Autodesk Inventor part; units mm, degrees
ref_plane "YZ Plane" through (0, 0, 0) normal (1, 0, 0) x (0, 1, 0)
ref_plane "XZ Plane" through (0, 0, 0) normal (0, 1, 0) x (-1, 0, 0)
ref_plane "XY Plane" through (0, 0, 0) normal (0, 0, 1) x (1, 0, 0)
sketch "Sketch1" plane through (0, 0, 0) normal (0, 1, 0) x (-1, 0, 0)
  circle A0 centre (0, 0) radius 50
  circle A1 centre (0, 0) radius 40
  line L0 (50, 0) -> (-50, 0)
  line L1 (-50, 0) -> (-50, 50)
  line L2 (-50, 50) -> (50, 50)
  line L3 (50, 50) -> (50, 0)
  line L4 (6, -46) -> (-6, -46)
  line L5 (-6, -46) -> (-6, -62)
  line L6 (-6, -62) -> (6, -62)
  line L7 (6, -62) -> (6, -46)
  line L8 (1, -64) -> (-1, -64)
  line L9 (-1, -64) -> (-1, -35)
  line L10 (-1, -35) -> (1, -35)
  line L11 (1, -35) -> (1, -64)
  point P0 (1, -39.9875)
  point P1 (1, -62)
  point P2 (6, -49.6387)
  point P3 (-6, -49.6387)
  point P4 (-1, -62)
  point P5 (-1, -39.9875)
  dimension "d0" = 100
extrude "Extrusion1" add sketch "Sketch1" along normal blind 70 contours L0 A1 A0 | A0 L7 L4 L11 A1 L0 | A0 L2 L3 | A0 L1 L2 | L7 L6 L11 A0 | A0 L11 L4 L7 | L0 A1 L9 L4 L5 A0 | L5 L4 L9 A0 | A0 L9 L6 L5
sketch "Sketch2" plane through (0, 70, 0) normal (0, 1, 0) x (1, 0, 0)
  circle A0 centre (0, 62) radius 3.05
  dimension "d9" = 6.1
extrude "Extrusion2" cut sketch "Sketch2" against normal blind 100
sketch "Sketch3" plane through (0, 70, 0) normal (0, 1, 0) x (1, 0, 0)
  line L0 (-3.05, 48) -> (-8, 48)
  line L1 (-8, 48) -> (-8, 62.2274)
  line L2 (-8, 62.2274) -> (-3.05, 62.2274)
  line L3 (-3.05, 62.2274) -> (-3.05, 48)
  line L4 (3.0501, 48) -> (8, 48)
  line L5 (8, 48) -> (8, 62.2274)
  line L6 (8, 62.2274) -> (3.0501, 62.2274)
  line L7 (3.0501, 62.2274) -> (3.0501, 48)
extrude "Extrusion3" add sketch "Sketch3" against normal up to surface (70 mm away)
sketch "Sketch4" plane through (0, 70, 0) normal (0, 1, 0) x (1, 0, 0)
  line L0 (8, 62.2274) -> (3.0501, 62.2274) construction
  line L1 (-3.05, 62.2274) -> (-8, 62.2274) construction
  arc A0 (-8, 49.3559) -> (-50, 0) centre (0, 0) ccw construction
  arc A1 (50, 0) -> (8, 49.3559) centre (0, 0) ccw construction
  line L2 (-8, 62.2274) -> (-20.0044, 45.8238)
  line L3 (8, 62.2274) -> (20.0044, 45.8238)
  line L4 (-20.0044, 45.8238) -> (-5.525, 45.8238)
  line L5 (-5.525, 45.8238) -> (-5.525, 62.2274)
  line L6 (-8, 62.2274) -> (-5.525, 62.2274)
  line L7 (20.0044, 45.8238) -> (5.5251, 45.8238)
  line L8 (5.5251, 45.8238) -> (5.5251, 62.2274)
  line L9 (5.5251, 62.2274) -> (8, 62.2274)
extrude "Extrusion4" add sketch "Sketch4" against normal blind 6
sketch "Sketch5" plane through (-50, 0, 50) normal (0, 0, 1) x (1, 0, 0)
  line L0 (46.95, 70) -> (46.95, 0) construction
  line L1 (0, 0) -> (100, 0) construction
  line L2 (100, 0) -> (100, 70) construction
  line L3 (0, 70) -> (100, 70) construction
  line L4 (0, 0) -> (0, 70) construction
  line L5 (0, 0) -> (100, 0)
  line L6 (100, 0) -> (100, 70)
  line L7 (100, 70) -> (0, 70)
  line L8 (0, 70) -> (0, 0)
  point P0 (50, 0)
extrude "Extrusion5" add sketch "Sketch5" along normal blind 10
properties part number "MotorClamp"
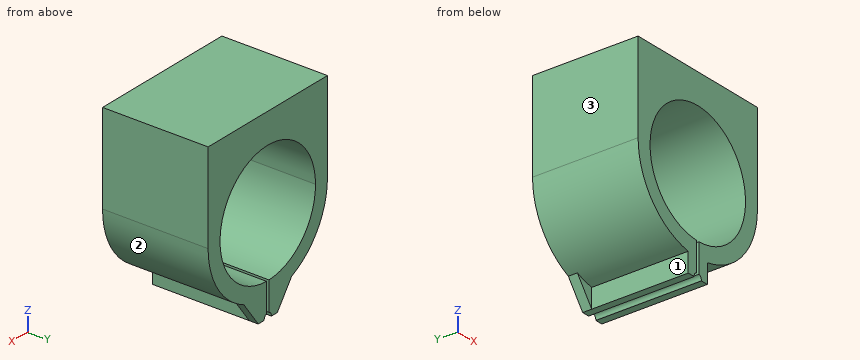
Check sheet for the modelled part. Datum: model origin and axes. Units: mm. Face numbers are marked on the shaded views. A direction names the side the tool comes from. Give positions to 0.01 mm unless a question says otherwise; leave off trailing zeros. Write each loop counter-clockwise with the first axis right and the second up, starting at its lowest first coordinate (ties: lowest second). Pieces come first, ordered by that corner, then holes. Notation, with made-up numbers: (-14, -0.75) - (8, -0.75) arc R9 ccw to (8, 11.25) - close; hole circle Ø11 at (-37.5, -12.5). An arc over 180 degrees is marked (long way). Answer as a JSON object with one key per item and string values. Group by question number.
1) Sectioned sample at B-B (z = 34). Record the cut outline in (x, y).
2) Sectioned sample at A-A (x = 24.5). Record the cut outline in (y, z), then the cut area to 3 significant figures.
3) Sectioned sample at D-D (x = -16). Record the cut outline in (y, z), then the cut area to 3 significant figures.
4) Depth check by flat-ended pin: P1, Ø10, axis at y = 25, z = -35, coming from the -X side; P2, Ø21, axis at y = 21.5, z = -46.5, coming from the +X side; P3, Ø15.5, axis at y = 51.5, z = -54, coming from the -X side. Enter the tip coordinate at first touch or a pass-through.
5) Sectioned sample at C-C (y = 18.5). Record the cut outline in (x, z), then the cut area to 3 significant figures.
6) Thickness scan on probe 1 along X at (y, z) = (16, 0); probe 2 along X at (y, z) = (12.5, -51.5); probe 3 along Z at (x, y) = (0, 40). Record the ranges inside material, lowest first. Write a range as from..to.
7) Access from +Z, -Z, +X, -X, +Y, -Y to the whole of each face (thin tool, end or side, straight path). Record for the marked faces 1, 2 and 3.
Geometry results:
{
 "1": {"outline": "(-50, 0) - (-21.07, 0) - (-21.07, 70) - (-50, 70) - close; (21.07, 0) - (50, 0) - (50, 70) - (21.07, 70) - close"},
 "2": {"outline": "(0, -43.59) - (70, -43.59) - (70, -31.62) - (0, -31.62) - close; (0, 31.62) - (70, 31.62) - (70, 60) - (0, 60) - close", "area": "2,820 mm^2"},
 "3": {"outline": "(0, -47.37) - (64, -47.37) - (64, -51.3) - (70, -51.3) - (70, -36.66) - (0, -36.66) - close; (0, 36.66) - (70, 36.66) - (70, 60) - (0, 60) - close", "area": "2,410 mm^2"},
 "4": {"P1": "stops at x = -40", "P2": "stops at x = 34.7", "P3": "stops at x = -19"},
 "5": {"outline": "(-50, 0) arc R50 ccw to (-8, -49.36) - (-8, -62.23) - (-3.05, -62.23) - (-3.05, -62) arc R3.05 cw to (-1, -59.12) - (-1, -39.99) arc R40 cw (long way) to (1, -39.99) - (1, -59.12) arc R3.05 cw to (3.05, -62) - (3.05, -62.23) - (8, -62.23) - (8, -49.36) arc R50 ccw to (50, 0) - (50, 60) - (-50, 60) - close", "area": "5,050 mm^2"},
 "6": {"probe 1": "x = -50..-40, 40..50", "probe 2": "x = -8..-1, 1..8", "probe 3": "z = 40..60"},
 "7": {"face 1": "-Z, -X, -Y", "face 2": "-Z, +X, -Y", "face 3": "+Z, -Z, -X, +Y, -Y"}
}
